Build history of the part. All positions in model axes, mm. Round coordinates to 2 decimals unless told otherwise and drop trailing zeros. Write each loop counter-clockwise with the first axis right and the second up, starting at its lowest first coordinate (ties: lowest second). Pieces come first, ordered by that corner, then holes.
Item 1: Drop flat-ended pins along their axis: pin 1 Ø5 at (x, z) = (26, 3) entering from -Y; pin 2 Ø2 at (x, z) = (-68, 2) entering from -Y; pin 3 Ø1 at (y, z) = (69.5, 4.5) entering from -X. Give the stop position or say it passes through.
Item 2: Band-saw the part on C-C, the plane z = 7. Write the cut outline in (x, y), then the cut area to 3 significant figures.
Item 3: Wall check: probe 1 along Y at (x, z) = (0, 1.55); probe 2 along Z at (x, y) = (-75, -49); probe 3 along Y at (x, z) = (-33, 6.25). Give the ranges that are in metal, low to high.
Item 4: Band-saw the part on A-A, the plane x = 0. Write the cut outline in (y, z), then the cut area to 3 significant figures.
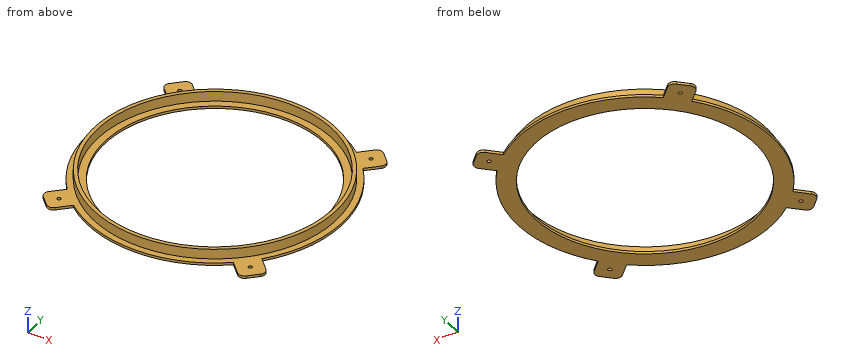
```python
from build123d import *

# Parameters (mm, degrees)
SKETCH_R        = 102.5
SKETCH_R_2      = 88.5
PAD_DEPTH       = 2
SKETCH001_R     = 97.5
SKETCH001_R_2   = 94.5
PAD001_DEPTH    = 8
PAD002_DEPTH    = 2
PAD003_DEPTH    = 2
SKETCH004_R     = 1.5
POCKET_DEPTH    = 2
SKETCH005_R     = 88.5
POCKET001_DEPTH = 2
FILLET_R        = 5
FILLET001_R     = 5
FILLET002_R     = 5
FILLET003_R     = 5


with BuildPart() as part:
    # Sketch → Pad (new body)
    with BuildSketch(Plane.XY):
        Circle(SKETCH_R)
        Circle(SKETCH_R_2, mode=Mode.SUBTRACT)
    extrude(amount=PAD_DEPTH)

    # Sketch001 (on Face4 of Pad) → Pad001 (join)
    with BuildSketch(Plane.XY.offset(2)):
        Circle(SKETCH001_R)
        Circle(SKETCH001_R_2, mode=Mode.SUBTRACT)
    extrude(amount=PAD001_DEPTH)

    # Sketch002 → Pad002 (join)
    with BuildSketch(Plane.XY):
        Polygon((-91.923836, 77.781784), (-77.781703, 91.923922), (91.923897, -77.781733), (77.781764, -91.923871), align=None)
    extrude(amount=PAD002_DEPTH)

    # Sketch003 → Pad003 (join)
    with BuildSketch(Plane.XY):
        Polygon((77.781763, 91.923871), (91.923897, 77.781733), (-77.781703, -91.923922), (-91.923836, -77.781784), align=None)
    extrude(amount=PAD003_DEPTH)

    # Sketch004 (on Face30 of Pad003) → Pocket (cut)
    with BuildSketch(Plane.XY.offset(2)):
        with Locations((77.781762, -77.781734)):
            Circle(SKETCH004_R)
        with Locations((-77.781701, -77.781785)):
            Circle(SKETCH004_R)
        with Locations((-77.781701, 77.781785)):
            Circle(SKETCH004_R)
        with Locations((77.781762, 77.781734)):
            Circle(SKETCH004_R)
    extrude(amount=-POCKET_DEPTH, mode=Mode.SUBTRACT)

    # Sketch005 (on Face36 of Pocket) → Pocket001 (cut)
    with BuildSketch(Plane.XY.offset(2)):
        Circle(SKETCH005_R)
    extrude(amount=-POCKET001_DEPTH, mode=Mode.SUBTRACT)

    # Fillet
    fillet_edges = [part.edges().sort_by_distance(p)[0] for p in [
        (91.923897, -77.781733, 1),
        (77.781764, -91.923871, 1),
    ]]
    fillet(fillet_edges, radius=FILLET_R)

    # Fillet001
    fillet001_edges = [part.edges().sort_by_distance(p)[0] for p in [
        (-77.781703, -91.923922, 1),
    ]]
    fillet(fillet001_edges, radius=FILLET001_R)

    # Fillet002
    fillet002_edges = [part.edges().sort_by_distance(p)[0] for p in [
        (-91.923836, -77.781784, 1),
    ]]
    fillet(fillet002_edges, radius=FILLET002_R)

    # Fillet003
    fillet003_edges = [part.edges().sort_by_distance(p)[0] for p in [
        (91.923897, 77.781733, 1),
        (77.781763, 91.923871, 1),
        (-77.781703, 91.923922, 1),
        (-91.923836, 77.781784, 1),
    ]]
    fillet(fillet003_edges, radius=FILLET003_R)


solid = part.part
```
Results:
1. pin 1: stops at y = -99.72
1. pin 2: stops at y = -83.14
1. pin 3: stops at x = -68.89
2. outline: circle Ø195 at (0, 0); hole circle Ø189 at (0, 0)
2. area: 1,810 mm2
3. probe 1: y = -102.5 to -88.5, 88.5 to 102.5
3. probe 2: z = 0 to 2
3. probe 3: y = -91.75 to -88.55, 88.55 to 91.75
4. outline: (-102.5, 0) - (-88.5, 0) - (-88.5, 2) - (-94.5, 2) - (-94.5, 10) - (-97.5, 10) - (-97.5, 2) - (-102.5, 2) - close; (88.5, 0) - (102.5, 0) - (102.5, 2) - (97.5, 2) - (97.5, 10) - (94.5, 10) - (94.5, 2) - (88.5, 2) - close
4. area: 104 mm2
